Part model, mm, in its own coordinate system. A direction names the side the tool comes from. Round coordinates to 2 decimals unless told otherwise and drop trailing zeros. Loops run counter-clockwise (first coordinate to the right, second up) from the corner with the lowest first, then second, coordinate; pieces in that order, holes last.
from build123d import *

# Parameters (mm, degrees)
BOSS_EXTRUDE1_DEPTH = 127
BOSS_EXTRUDE4_DEPTH = 127
SKETCH7_R           = 1.375
SKETCH7_R_2         = 1.375000009
SKETCH7_R_3         = 1.374999997
SKETCH7_W           = 3.5
SKETCH7_H           = 7.028015283
SKETCH7_W_2         = 6.780603604
SKETCH7_H_2         = 3.5
SKETCH7_H_3         = 6.780603604
CUT_EXTRUDE2_DEPTH  = 131.426224357
SKETCH8_W           = 2.834613859
SKETCH8_H           = 1
SKETCH8_W_2         = 1
SKETCH8_H_2         = 2.748258962
SKETCH8_W_3         = 3.182807673
SKETCH8_H_3         = 2.560440129
CUT_EXTRUDE3_DEPTH  = 131.426224357
FILLET3_R           = 0.5
FILLET4_R           = 0.5
BOSS_EXTRUDE6_DEPTH = 127
FILLET5_R           = 6


# Some blends are built 0.0001 mm under size
with BuildPart() as part:
    # Sketch1 → Boss-Extrude1 (new body)
    with BuildSketch(Plane.XY):
        Polygon((4.990301802, 16.842973424), (16.842973424, 4.990301802), (16.842973424, -4.990301802), (4.990301802, -16.842973424), (-4.990301802, -16.842973424), (-16.842973424, -4.990301802), (-16.842973424, 4.990301802), (-4.990301802, 16.842973424), align=None)
        with BuildLine():
            Line((-13.745064738, 5.259783364), (-5.259783364, 13.745064738))
            ThreePointArc((-5.259783364, 13.745064738), (0, 11.566391134), (5.259783364, 13.745064738))
            Line((5.259783364, 13.745064738), (13.745064738, 5.259783364))
            ThreePointArc((13.745064738, 5.259783364), (11.566391134, 0), (13.745064738, -5.259783364))
            Line((13.745064738, -5.259783364), (5.259783364, -13.745064738))
            ThreePointArc((5.259783364, -13.745064738), (0, -11.566391134), (-5.259783364, -13.745064738))
            Line((-5.259783364, -13.745064738), (-13.745064738, -5.259783364))
            ThreePointArc((-13.745064738, -5.259783364), (-11.566391134, 0), (-13.745064738, 5.259783364))
        make_face(mode=Mode.SUBTRACT)
    extrude(amount=BOSS_EXTRUDE1_DEPTH)

    # Sketch5 → Boss-Extrude4 (add, through all)
    with BuildSketch(Plane.XY.offset(127)):
        Polygon((-16.842973424, -4.990301802), (-21, -4.990301802), (-21, -2.140301802), (-20, -2.140301802), (-20, -3.513722258), (-16.842973424, -3.513722258), align=None)
        Polygon((-16.842973424, 4.990301802), (-21, 4.990301802), (-21, 2.140301802), (-20, 2.140301802), (-20, 3.514293025), (-16.842973424, 3.514293025), align=None)
        Polygon((16.842973424, 4.990301802), (21, 4.990301802), (21, 2.140301802), (20, 2.140301802), (20, 3.390301802), (16.842973424, 3.390301802), align=None)
        Polygon((21, -4.990301802), (16.842973424, -4.990301802), (16.842973424, -3.390301802), (20, -3.390301802), (20, -2.140301802), (21, -2.140301802), align=None)
        Polygon((3.390301802, 16.842973424), (4.990301802, 16.842973424), (4.990301802, 21), (2.140301802, 21), (2.140301802, 20), (3.390301802, 20), align=None)
        Polygon((-4.990301802, 16.842973424), (-4.990301802, 21), (-2.140301802, 21), (-2.140301802, 20), (-3.390301802, 20), (-3.390301802, 16.842973424), align=None)
        Polygon((4.990301802, -16.842973424), (4.990301802, -21), (2.140301802, -21), (2.140301802, -20), (3.390301802, -20), (3.390301802, -16.842973424), align=None)
        Polygon((-4.990301802, -16.842973424), (-4.990301802, -21), (-2.140301802, -21), (-2.140301802, -20), (-3.390301802, -20), (-3.390301802, -16.842973424), align=None)
    extrude(amount=-BOSS_EXTRUDE4_DEPTH)

    # Sketch7 → Cut-Extrude2 (cut, through all)
    with BuildSketch(Plane.XY):
        with Locations(Location((-15.004848102, 0, 0), (0, 0, 180))):
            Circle(SKETCH7_R)
        with Locations(Location((3e-09, 15.004848102, 0), (0, 0, 180))):
            Circle(SKETCH7_R)
        with Locations(Location((15.004848102, -2.203e-06, 0), (0, 0, 180))):
            Circle(SKETCH7_R_2)
        with Locations(Location((0, -15.004848102, 0), (0, 0, 180))):
            Circle(SKETCH7_R_3)
        with Locations((-18.25, 0.000285384)):
            Rectangle(SKETCH7_W, SKETCH7_H)
        with Locations((0, 18.25)):
            Rectangle(SKETCH7_W_2, SKETCH7_H_2)
        with Locations((18.25, 0)):
            Rectangle(SKETCH7_W, SKETCH7_H_3)
        with Locations((0, -18.25)):
            Rectangle(SKETCH7_W_2, SKETCH7_H_2)
    extrude(amount=CUT_EXTRUDE2_DEPTH, mode=Mode.SUBTRACT)

    # Sketch8 → Cut-Extrude3 (cut, through all)
    with BuildSketch(Plane.XY.offset(127)):
        with Locations((-16.422155032, 0)):
            Rectangle(SKETCH8_W, SKETCH8_H)
        with Locations((0, 16.378977583)):
            Rectangle(SKETCH8_W_2, SKETCH8_H_2)
        with Locations((16.596251939, 0)):
            Rectangle(SKETCH8_W_3, SKETCH8_H)
        with Locations((0, -16.285068167)):
            Rectangle(SKETCH8_W_2, SKETCH8_H_3)
    extrude(amount=-CUT_EXTRUDE3_DEPTH, mode=Mode.SUBTRACT)

    # Fillet3
    # the kernel refuses this fillet: 0.5 mm, written as the material it takes off along each edge
    with BuildSketch(Plane(origin=(-16.5, 0.5, -1.025810125), x_dir=(0, 1, 0), z_dir=(0, 0, 1))) as fillet3_piece_1:
        with BuildLine():
            CenterArc((0.41032405, -0.5), FILLET3_R, 90, 55.149723763)
            Line((0, -0.214283053), (-0.008206481, -0.208568714))
            ThreePointArc((-0.008206481, -0.208568714), (-0.01, -0.107141526), (-0.01, 0))
            Line((-0.01, 0), (0, 0.01))
            Line((0, 0.01), (0.41032405, 0.01))
            Line((0.41032405, 0.01), (0.41032405, 0))
        make_face()
    extrude(amount=129.05162025, mode=Mode.SUBTRACT)
    with BuildSketch(Plane(origin=(0.5, -16.5, -1.02581013), x_dir=(5.296643708926083e-12, 1.0, 0), z_dir=(0, 0, 1))) as fillet3_piece_2:
        with BuildLine():
            CenterArc((0.5, -0.410324052), FILLET3_R, 124.850275833, 55.149724167)
            Line((0, -0.410324052), (-0.01, -0.410324052))
            Line((-0.01, -0.410324052), (-0.01, 0))
            Line((-0.01, 0), (0, 0.01))
            ThreePointArc((0, 0.01), (0.107141528, 0.01), (0.208568717, 0.008206481))
            Line((0.208568717, 0.008206481), (0.214283056, 0))
        make_face()
    extrude(amount=129.05162026, mode=Mode.SUBTRACT)
    with BuildSketch(Plane(origin=(-0.5, -16.5, 128.02581013), x_dir=(-1, 0, 0), z_dir=(0, 0, -1))) as fillet3_piece_3:
        with BuildLine():
            CenterArc((0.410324052, 0.5), FILLET3_R, 214.850275833, 55.149724167)
            Line((0, 0.214283056), (-0.008206481, 0.208568717))
            ThreePointArc((-0.008206481, 0.208568717), (-0.01, 0.107141528), (-0.01, 0))
            Line((-0.01, 0), (0, -0.01))
            Line((0, -0.01), (0.410324052, -0.01))
            Line((0.410324052, -0.01), (0.410324052, 0))
        make_face()
    extrude(amount=129.05162026, mode=Mode.SUBTRACT)
    with BuildSketch(Plane(origin=(16.5, -0.5, -1.025808612), x_dir=(0, -1, 0), z_dir=(0, 0, 1))) as fillet3_piece_4:
        with BuildLine():
            CenterArc((0.410323445, -0.5), FILLET3_R, 90, 55.149602377)
            Line((0, -0.214282183), (-0.008206469, -0.208567827))
            ThreePointArc((-0.008206469, -0.208567827), (-0.01, -0.107141092), (-0.01, 0))
            Line((-0.01, 0), (0, 0.01))
            Line((0, 0.01), (0.410323445, 0.01))
            Line((0.410323445, 0.01), (0.410323445, 0))
        make_face()
    extrude(amount=129.051617223, mode=Mode.SUBTRACT)
    with BuildSketch(Plane(origin=(16.5, 0.5, 128.025811605), x_dir=(-1.0, 5.295068435052625e-12, 0), z_dir=(0, 0, -1))) as fillet3_piece_5:
        with BuildLine():
            CenterArc((0.5, 0.410324642), FILLET3_R, 180, 55.149842509)
            Line((0, 0.410324642), (-0.01, 0.410324642))
            Line((-0.01, 0.410324642), (-0.01, 0))
            Line((-0.01, 0), (0, -0.01))
            ThreePointArc((0, -0.01), (0.107141952, -0.01), (0.208569581, -0.008206493))
            Line((0.208569581, -0.008206493), (0.214283903, 0))
        make_face()
    extrude(amount=129.051623211, mode=Mode.SUBTRACT)
    with BuildSketch(Plane(origin=(-0.5, 16.5, -1.025810127), x_dir=(-5.291980756940643e-12, -1.0, 0), z_dir=(0, 0, 1))) as fillet3_piece_6:
        with BuildLine():
            CenterArc((0.5, -0.410324051), FILLET3_R, 124.850276074, 55.149723926)
            Line((0, -0.410324051), (-0.01, -0.410324051))
            Line((-0.01, -0.410324051), (-0.01, 0))
            Line((-0.01, 0), (0, 0.01))
            ThreePointArc((0, 0.01), (0.107141527, 0.01), (0.208568715, 0.008206481))
            Line((0.208568715, 0.008206481), (0.214283054, 0))
        make_face()
    extrude(amount=129.051620254, mode=Mode.SUBTRACT)
    with BuildSketch(Plane(origin=(0.5, 16.5, 128.025810123), x_dir=(1, 0, 0), z_dir=(0, 0, -1))) as fillet3_piece_7:
        with BuildLine():
            CenterArc((0.410324049, 0.5), FILLET3_R, 214.8502764, 55.1497236)
            Line((0, 0.214283051), (-0.008206481, 0.208568713))
            ThreePointArc((-0.008206481, 0.208568713), (-0.01, 0.107141526), (-0.01, 0))
            Line((-0.01, 0), (0, -0.01))
            Line((0, -0.01), (0.410324049, -0.01))
            Line((0.410324049, -0.01), (0.410324049, 0))
        make_face()
    extrude(amount=129.051620246, mode=Mode.SUBTRACT)
    with BuildSketch(Plane(origin=(-16.5, -0.5, 128.025810125), x_dir=(1.0, -5.296125669893669e-12, 0), z_dir=(0, 0, -1))) as fillet3_piece_8:
        with BuildLine():
            CenterArc((0.5, 0.41032405), FILLET3_R, 180, 55.149723763)
            Line((0, 0.41032405), (-0.01, 0.41032405))
            Line((-0.01, 0.41032405), (-0.01, 0))
            Line((-0.01, 0), (0, -0.01))
            ThreePointArc((0, -0.01), (0.107141526, -0.01), (0.208568714, -0.008206481))
            Line((0.208568714, -0.008206481), (0.214283053, 0))
        make_face()
    extrude(amount=129.05162025, mode=Mode.SUBTRACT)

    # Fillet4
    fillet4_edges = [part.edges().sort_by_distance(p)[0] for p in [
        (-16.285716947, 0.5, 63.5),
        (0.5, -16.285716944, 63.5),
        (-0.5, -16.285716944, 63.5),
        (16.285717817, -0.5, 63.5),
        (16.285716097, 0.5, 63.5),
        (-0.5, 16.285716946, 63.5),
        (0.5, 16.285716949, 63.5),
        (-16.285716947, -0.5, 63.5),
    ]]
    fillet(fillet4_edges, radius=FILLET4_R - 0.0001)  # a hair under: the kernel refuses the full size

    # Sketch9 → Boss-Extrude6 (add, through all)
    with BuildSketch(Plane.XY.offset(127)):
        with BuildLine():
            Line((-4.990301802, 16.842973424), (-16.842973424, 4.990301802))
            ThreePointArc((-16.842973424, 4.990301802), (-11.852671623, 0), (-16.842973424, -4.990301802))
            Line((-16.842973424, -4.990301802), (-4.990301802, -16.842973424))
            ThreePointArc((-4.990301802, -16.842973424), (0, -11.852671623), (4.990301802, -16.842973424))
            Line((4.990301802, -16.842973424), (16.842973424, -4.990301802))
            ThreePointArc((16.842973424, -4.990301802), (11.852671623, 0), (16.842973424, 4.990301802))
            Line((16.842973424, 4.990301802), (4.990301802, 16.842973424))
            ThreePointArc((4.990301802, 16.842973424), (0, 11.852671623), (-4.990301802, 16.842973424))
        make_face()
        Polygon((-5.259783364, 13.745064738), (-13.745064738, 5.259783364), (-8.485281374, 0), (-13.745064738, -5.259783364), (-5.259783364, -13.745064738), (0, -8.485281374), (5.259783364, -13.745064738), (13.745064738, -5.259783364), (8.485281374, 0), (13.745064738, 5.259783364), (5.259783364, 13.745064738), (0, 8.485281374), align=None, mode=Mode.SUBTRACT)
    extrude(amount=-BOSS_EXTRUDE6_DEPTH)

    # Fillet5
    fillet5_edges = [part.edges().sort_by_distance(p)[0] for p in [
        (0, 8.485281374, 63.5),
        (8.485281374, 0, 63.5),
        (0, -8.485281374, 63.5),
        (-8.485281374, 0, 63.5),
    ]]
    fillet(fillet5_edges, radius=FILLET5_R)


solid = part.part
1) Slice it at A-A, the plane x = 18. Give the cut face in (y, z), then the cut area to 3 significant figures.
Values:
outline: (-4.99, 0) - (-3.39, 0) - (-3.39, 127) - (-4.99, 127) - close; (3.39, 0) - (4.99, 0) - (4.99, 127) - (3.39, 127) - close
area: 406 mm2
2) Wall check: line 1 along Y through (x, z) = (0, 87); line 2 along X through (y, z) = (3, 33); line 3 along Y through (x, z) = (-2.5, 114). Give the ranges that are in metal, low to high.
Values:
line 1: y = -13.63 to -10.97, 10.97 to 13.63
line 2: x = -21 to -20, -16.5 to -11.77, 11.77 to 16.5, 20 to 21
line 3: y = -21 to -20, -16.5 to -11.52, 11.52 to 16.5, 20 to 21
3) Mould opens along Y. For faces 1 (the face through (10.834, 11, 62.611)), 2 (the face through (-0.07, 10.97, 62.61)), 3 (the face through (19, -4.99, 64)) say: released by +Y, released by -Y, zero draft, split by the parting line, or undercut.
Values:
face 1: released by +Y
face 2: undercut
face 3: released by -Y
4) Drop flat-ended pins along their axis: pin 1 Ø3.5 at (x, z) = (-18.5, 73.5) entering from +Y; pin 2 Ø4.5 at (x, z) = (-19, 54) entering from -Y; pin 3 Ø3 at (x, z) = (-18, 72) entering from +Y. Give the stop position or say it passes through.
Values:
pin 1: stops at y = 5.08
pin 2: stops at y = -5.08
pin 3: stops at y = 5.33
5) Tool access for faces 4 (the face through (-4, 21, 64)), 5 (the face through (-19, 4.99, 64)), 6 (the face through (-3.39, 18, 63)): list every direction of +Z, -Z, +X, -X, +Y, -Y with a clear straight run to the whole face (end or side of a thin tool).
Values:
face 4: +Z, -Z, +X, -X, +Y
face 5: +Z, -Z, -X, +Y
face 6: +Z, -Z
